Verification items for the finished model (mm, model axes). A direction names the side the tool comes from. Coordinates: 2 decimals unless noted, no trailing zeros. Order: outer loops, then holes, each group sorted by start corner. A loop starts at its lowest first (then second) coordinate and runs counter-clockwise, first axis right, second up.
Q1. Thickness scan on line 1 (Z direction, x = -22, y = -5.5); line 2 (X direction, y = 0.5, z = 97.5); line 3 (Y direction, x = -10, z = 63). Record the ranges inside material, lowest first.
Q2. Cross-section at D-D, the plane y = -2.25. Record the boundary of the cut face in (x, z), and give its area (3 significant figures).
Q3. Depth check by flat-ended pin: P1, Ø2, axis at y = 2, z = 88, coming from the -X side; P2, Ø6, axis at x = -4.5, z = 58, coming from the -Y side; P3, Ø8, axis at x = -8.5, y = 3.5, coming from the +Z side; P4, Ø5, axis at y = -3, z = 95.5, coming from the -X side (3 decimals). Enter the tip coordinate at first touch or a pass-through.
Q4. Cross-section at C-C, the plane z = 89. Record the boundary of the cut face in (x, y), and give its area (4 significant figures).
Q5. Set-up check for faces 1 (the flat face through (15, 3, 85)), 2 (the flat face through (0, -4, 55)), 3 (the flat face through (0, 4, 95)), 4 (the flat face through (7, -4, 60)): record each of +Z, -Z, +X, -X, +Y, -Y from which the full face is reachable in a straight line by a thin tool's end or side.
Q6. Cross-section at A-A, the plane y = 6. Record the boundary of the cut face in (x, z), and give its area (3 significant figures).
Q7. Cross-section at B-B, the plane x = -9. Record the boundary of the cut face in (y, z), and give its area (3 significant figures).
from build123d import *

# Parameters (mm, degrees)
SKETCH_1_W               = 50
SKETCH_1_H               = 15
EXTRUDE_1_DEPTH          = 60
SKETCH_2_W               = 15
SKETCH_2_H               = 15
EXTRUDE_2_DEPTH          = 60
SKETCH_3_W               = 15
SKETCH_3_H               = 7.5
CUT_EXTRUDE_1_DEPTH      = 60
CUT_EXTRUDE_2_DEPTH      = 10
SKETCH_6_W               = 10
SKETCH_6_H               = 10
SKETCH_6_W_2             = 25
CUT_EXTRUDE_3_DEPTH      = 20
EXTRUDE_3_DEPTH          = 7.5
CUT_EXTRUDE_4_DEPTH      = 124.490890352
CUT_EXTRUDE_4_DEPTH_BACK = 124.490890352
SKETCH_7_W               = 82.157848782
SKETCH_7_H               = 26


with BuildPart() as part:
    # 스케치1 → 보스-돌출1 (new body)
    with BuildSketch(Plane.XY):
        Rectangle(SKETCH_1_W, SKETCH_1_H)
    extrude(amount=EXTRUDE_1_DEPTH)

    # 스케치2 → 보스-돌출2 (add)
    with BuildSketch(Plane.XY.offset(60)):
        with Locations((7.5, 0)):
            Rectangle(SKETCH_2_W, SKETCH_2_H)
    extrude(amount=EXTRUDE_2_DEPTH)

    # 스케치3 → 컷-돌출1 (cut)
    with BuildSketch(Plane.XY.offset(120)):
        with Locations((7.5, -3.75)):
            Rectangle(SKETCH_3_W, SKETCH_3_H)
    extrude(amount=-CUT_EXTRUDE_1_DEPTH, mode=Mode.SUBTRACT)

    # 스케치4 → 컷-돌출2 (cut)
    with BuildSketch(Plane(origin=(0, 7.5, 0), x_dir=(1, 0, 0), z_dir=(0, 1, 0))):
        with BuildLine():
            Line((0, -110), (0, -120))
            Line((0, -120), (10, -120))
            ThreePointArc((10, -120), (7.071067812, -112.928932188), (0, -110))
        make_face()
    extrude(amount=-CUT_EXTRUDE_2_DEPTH, mode=Mode.SUBTRACT)

    # 스케치6 → 컷-돌출3 (cut)
    with BuildSketch(Plane(origin=(0, 7.5, 0), x_dir=(1, 0, 0), z_dir=(0, 1, 0))):
        with Locations((20, -55)):
            Rectangle(SKETCH_6_W, SKETCH_6_H)
        with Locations((-12.5, -55)):
            Rectangle(SKETCH_6_W_2, SKETCH_6_H)
    extrude(amount=-CUT_EXTRUDE_3_DEPTH, mode=Mode.SUBTRACT)

    # 스케치5 → 보스-돌출3 (add)
    with BuildSketch(Plane(origin=(0, 7.5, 0), x_dir=(1, 0, 0), z_dir=(0, 1, 0))):
        Polygon((0, -50), (0, -80), (-20, -50), align=None)
    extrude(amount=-EXTRUDE_3_DEPTH)

    # 스케치7 → 컷-돌출4 (cut, two sides: drawn at the far end of the back side and taken through both)
    with BuildSketch(Plane.XZ.offset(7.5).offset(-CUT_EXTRUDE_4_DEPTH_BACK)):
        Rectangle(SKETCH_7_W, SKETCH_7_H)
    extrude(amount=CUT_EXTRUDE_4_DEPTH + CUT_EXTRUDE_4_DEPTH_BACK, mode=Mode.SUBTRACT)


solid = part.part
Check values:
1. line 1: z = 13 to 50
1. line 2: x = 0 to 15
1. line 3: y = 0 to 7.5
2. outline: (-25, 13) - (25, 13) - (25, 50) - (15, 50) - (15, 60) - (0, 60) - (0, 50) - (-25, 50) - close
2. area: 2,000 mm2
3. P1: stops at x = 0
3. P2: stops at y = 0
3. P3: stops at z = 73.25
3. P4: passes through
4. outline: (0, 0) - (15, 0) - (15, 7.5) - (0, 7.5) - close
4. area: 112.5 mm2
5. face 1: +Z, +X, +Y, -Y
5. face 2: +Z, -X, -Y
5. face 3: +Z, -X, +Y, -Y
5. face 4: +Z, +X, -X, -Y
6. outline: (-25, 13) - (25, 13) - (25, 50) - (15, 50) - (15, 120) - (10, 120) arc R10 cw to (0, 110) - (0, 80) - (-20, 50) - (-25, 50) - close
6. area: 3,120 mm2
7. outline: (-7.5, 13) - (7.5, 13) - (7.5, 66.5) - (0, 66.5) - (0, 50) - (-7.5, 50) - close
7. area: 679 mm2
